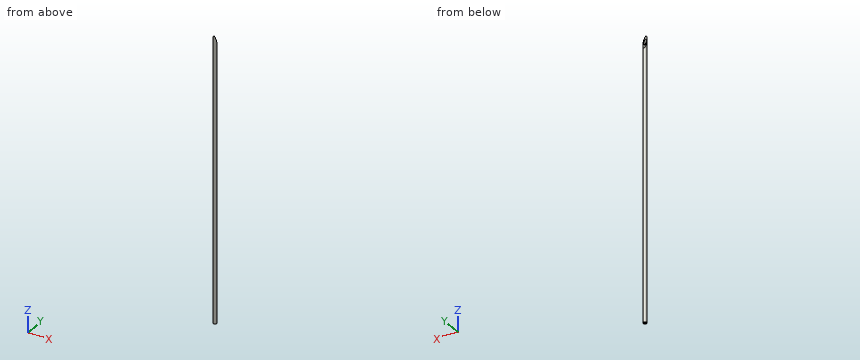
Autodesk Inventor part; units mm, degrees
ref_plane "YZ Plane" through (0, 0, 0) normal (1, 0, 0) x (0, 1, 0)
ref_plane "XZ Plane" through (0, 0, 0) normal (0, 1, 0) x (-1, 0, 0)
ref_plane "XY Plane" through (0, 0, 0) normal (0, 0, 1) x (1, 0, 0)
sketch "Sketch1" plane through (0, 0, 0) normal (0, 0, 1) x (1, 0, 0)
  circle A0 centre (0, 0) radius 0.205
  dimension "d0" = 0.41
extrude "Extrusion5" add sketch "Sketch1" along normal blind 31.7
hole "Hole2" at (0, 0, 0) direction (0, 0, 1) diameter 0.2 end through all
sketch "Sketch10" plane through (0, 0, 0) normal (1, 0, 0) x (0, 1, 0)
  line L0 (0, -6.34) -> (0, 38.04)
  line L1 (-0.205, 31.7) -> (0.205, 31.7)
  line L2 (0.205, 0) -> (0.205, 31.7)
  line L3 (-0.205, 31.7) -> (0.205, 30.1699)
  line L4 (0.205, 31.7) -> (-0.205, 31.7)
  line L5 (0.205, 30.1699) -> (0.205, 31.7)
  point P0 (0, 0)
  dimension "d52" = 15
  dimension "d53" = 1.5301
extrude "Extrusion6" cut sketch "Sketch10" along normal through all both and the other way through all
properties part number "Needle"
Input: part model. Units: mm. Frame: model coordinates. Coordinates: 2 decimals unless noted, no trailing zeros. Order: outer loops, then holes, each group sorted by start corner. A loop starts at its lowest first (then second) coordinate and runs counter-clockwise, first axis right, second up. Notation, with made-up numbers: M 43.25,41.25 L 87.25,41.25 A4 ccw 87.25,46.25 Z; hole C 77.25,-39.5 d3. An arc over 180 degrees is marked long. Answer in a Markdown table with one row per item.
(1) Material intervals for line 1 (Y direction, x = 0.15, z = 2.5), sorted ascending. Write a range as [from, to].
Numbers:
| item | result |
|---|---|
| line 1 | y = [-0.14, 0.14] |
(2) Section query A-A, the plane x = 0. Output: boundary loops of the cut face in (y, z) (3 decimals).
Numbers:
| item | result |
|---|---|
| outline | M -0.205,0 L -0.1,0 L -0.1,31.308 L -0.205,31.7 Z; M 0.1,0 L 0.205,0 L 0.205,30.17 L 0.1,30.562 Z |
(3) Section query B-B, the plane z = 6. Output: boundary loops of the cut face in (x, y) (3 decimals), plus the area to 3 significant figures.
Numbers:
| item | result |
|---|---|
| outline | C 0,0 d0.41; hole C 0,0 d0.2 |
| area | 0.101 mm^2 |
